```python
from build123d import *

# Parameters (mm, degrees)
ESQUISSE1_W             = 247
ESQUISSE1_H             = 247
ESQUISSE1_R             = 12.5
ESQUISSE1_R_2           = 6.5
BOSS_EXTRU_1_DEPTH      = 3
CONG_1_R                = 30
ENL_V_MAT_EXTRU_2_DEPTH = 10


with BuildPart() as part:
    # Esquisse1 → Boss.-Extru.1 (new body)
    with BuildSketch(Plane.XY):
        Rectangle(ESQUISSE1_W, ESQUISSE1_H)
        with Locations((76.5, 41.5)):
            Circle(ESQUISSE1_R, mode=Mode.SUBTRACT)
        with Locations((76.5, 86.5)):
            Circle(ESQUISSE1_R_2, mode=Mode.SUBTRACT)
        with Locations((76.5, -3.5)):
            Circle(ESQUISSE1_R_2, mode=Mode.SUBTRACT)
    extrude(amount=BOSS_EXTRU_1_DEPTH)

    # Congé1
    cong_1_edges = [part.edges().sort_by_distance(p)[0] for p in [
        (123.5, -123.5, 1.5),
    ]]
    fillet(cong_1_edges, radius=CONG_1_R)

    # Esquisse4 → Enlèv. mat.-Extru.2 (cut)
    with BuildSketch(Plane(origin=(0, 0, 0), x_dir=(-1, 0, 0), z_dir=(0, 0, -1))):
        with BuildLine():
            Line((-83, 79), (-83, 94))
            ThreePointArc((-83, 94), (-76.5, 100.5), (-70, 94))
            Line((-70, 94), (-70, 79))
            ThreePointArc((-70, 79), (-76.5, 72.5), (-83, 79))
        make_face()
        with BuildLine():
            Line((-83, -11), (-83, 4))
            ThreePointArc((-83, 4), (-76.5, 10.5), (-70, 4))
            Line((-70, 4), (-70, -11))
            ThreePointArc((-70, -11), (-76.5, -17.5), (-83, -11))
        make_face()
        with BuildLine():
            Line((-89, 34), (-89, 49))
            ThreePointArc((-89, 49), (-76.5, 61.5), (-64, 49))
            Line((-64, 49), (-64, 34))
            ThreePointArc((-64, 34), (-76.5, 21.5), (-89, 34))
        make_face()
    extrude(amount=-ENL_V_MAT_EXTRU_2_DEPTH, mode=Mode.SUBTRACT)


solid = part.part
```
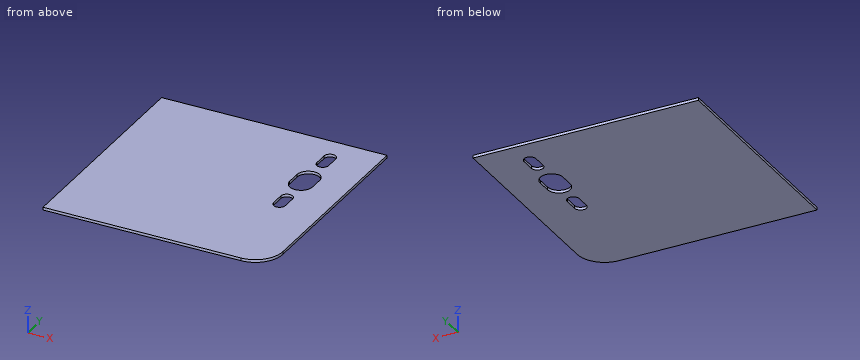
The model under review builds one solid part; all positions refer to its coordinate system, in mm. Round coordinates to 2 decimals unless told otherwise and drop trailing zeros. Loops run counter-clockwise (first coordinate to the right, second up) from the corner with the lowest first, then second, coordinate; pieces in that order, holes last.
Item 1: Take a section at B-B (x = 76.5). Write out the cut boundary in (y, z).
Determined:
outline: (-123.5, 0) - (-17.5, 0) - (-17.5, 3) - (-123.5, 3) - close; (10.5, 0) - (21.5, 0) - (21.5, 3) - (10.5, 3) - close; (61.5, 0) - (72.5, 0) - (72.5, 3) - (61.5, 3) - close; (100.5, 0) - (123.5, 0) - (123.5, 3) - (100.5, 3) - close
Item 2: Take a section at A-A (z = 2.5). Write out the cut boundary in (x, y).
Determined:
outline: (-123.5, -123.5) - (93.5, -123.5) arc R30 ccw to (123.5, -93.5) - (123.5, 123.5) - (-123.5, 123.5) - close; hole (64, 34) arc R12.5 ccw to (89, 34) - (89, 49) arc R12.5 ccw to (64, 49) - close; hole (70, -11) arc R6.5 ccw to (83, -11) - (83, 4) arc R6.5 ccw to (70, 4) - close; hole (70, 79) arc R6.5 ccw to (83, 79) - (83, 94) arc R6.5 ccw to (70, 94) - close
Item 3: For line 1 (Y direction, x = 76.5, z = 0.55); line 2 (X direction, y = 94.5, z = 1.9); line 3 (Y direction, x = 81, z = 0.3), list the stretches that pass through material, from the lowest coordinate up.
Determined:
line 1: y = -123.5 to -17.5, 10.5 to 21.5, 61.5 to 72.5, 100.5 to 123.5
line 2: x = -123.5 to 70.02, 82.98 to 123.5
line 3: y = -123.5 to -15.69, 8.69 to 22.34, 60.66 to 74.31, 98.69 to 123.5
